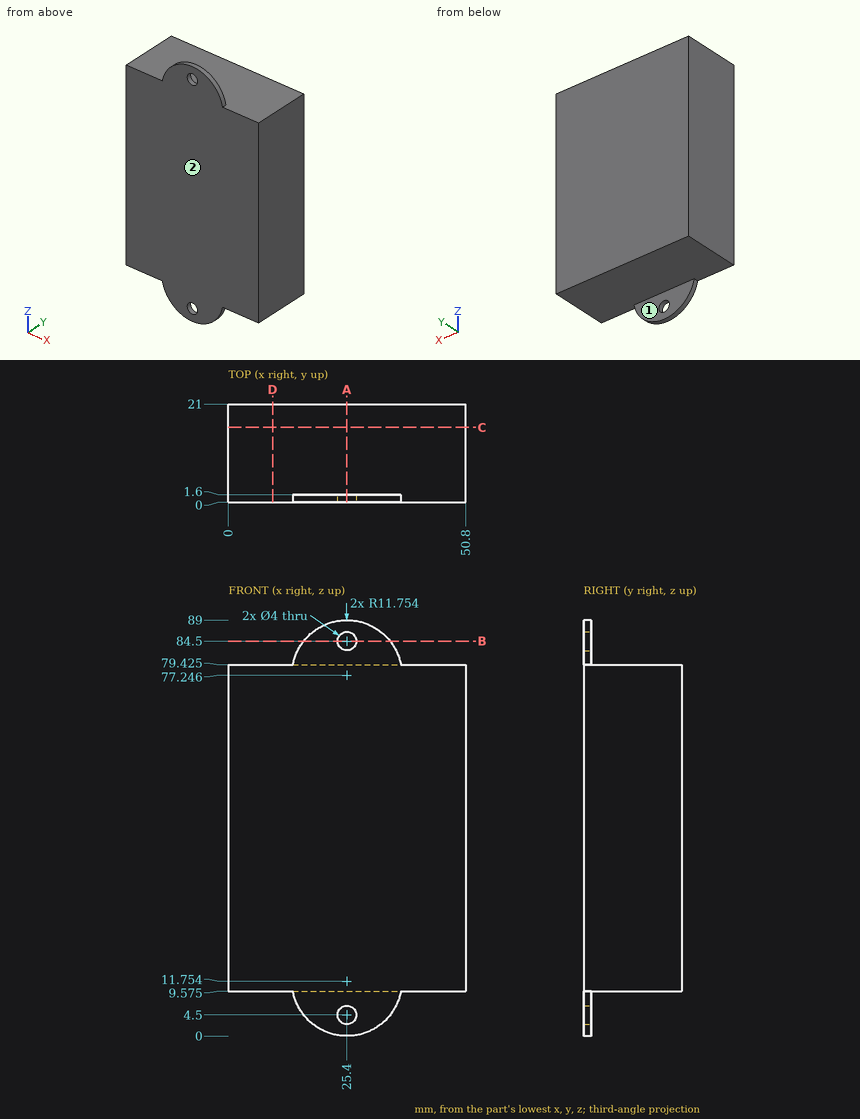
Study the drawing (mm; zero at the part's minimum x, y, z) and answer. A direction names the side the tool comes from. Coordinates: 2 decimals unless noted, no trailing zeros. Loops run counter-clockwise (first coordinate to the right, second up) from the corner with the lowest first, then second, coordinate; pieces in that order, holes last. Notation, with made-up numbers: (17.5, 68) -> (47.5, 68) arc R20 cw to (47.5, 99) -> close; hole circle Ø11 at (2, 68). An arc over 180 degrees is marked (long way). Answer as CSV lines item,"result".
1) The part is cut by section D-D (x = 9.5). Give the vertices of the cut face in (y, z) (1 decimal).
A:
outline,"(0, 9.6) -> (21, 9.6) -> (21, 79.4) -> (0, 79.4) -> close"
2) The part is cut by section C-C (y = 16). Give the vertices of the cut face in (x, z) (1 decimal).
A:
outline,"(0, 9.6) -> (50.8, 9.6) -> (50.8, 79.4) -> (0, 79.4) -> close"
3) Straight lines are drawn through the part: probe 1 along Z at (x, y) = (25.4, 0.9); probe 2 along Z at (x, y) = (46, 8) (1 decimal); probe 3 along X at (y, z) = (0.4, 84.5). For each, find the intervals that lie inside material, in ascending order.
A:
probe 1,"z = 0 to 2.5, 6.5 to 82.5, 86.5 to 89"
probe 2,"z = 9.6 to 79.4"
probe 3,"x = 16.15 to 23.4, 27.4 to 34.65"
4) The part is cut by section A-A (x = 25.4). Give the vertices of the cut face in (y, z) (1 decimal).
A:
outline,"(0, 0) -> (1.6, 0) -> (1.6, 2.5) -> (0, 2.5) -> close; (0, 6.5) -> (1.6, 6.5) -> (1.6, 9.6) -> (21, 9.6) -> (21, 79.4) -> (1.6, 79.4) -> (1.6, 82.5) -> (0, 82.5) -> close; (0, 86.5) -> (1.6, 86.5) -> (1.6, 89) -> (0, 89) -> close"
5) For the marked faces 1 and 2, determine the directions among +Z, -Z, +X, -X, +Y, -Y from which every point of the face is accessible in a straight line to the end or side of a thin tool.
A:
face 1,"-Z, +X, -X, +Y"
face 2,"+Z, -Z, +X, -X, -Y"
6) The part is cut by section B-B (z = 84.5). Give the vertices of the cut face in (x, y), and give its area (3 significant figures).
A:
outline,"(16.15, 0) -> (23.4, 0) -> (23.4, 1.6) -> (16.15, 1.6) -> close; (27.4, 0) -> (34.65, 0) -> (34.65, 1.6) -> (27.4, 1.6) -> close"
area,"23.2 mm²"
7) Flat-ended cylindrical pins translate along their axes: pin 1 (1 mm diameter, centred on x = 7.5, y = 12, fed in from +Z) (3 decimals); pin 2 (8 mm diameter, centred on x = 14.5, y = 2.5, fed in from +Z); pin 3 (5 mm diameter, centred on x = 26, z = 82.5, fed in from +Y). Find the tip coordinate at first contact, or state that the pin passes through.
A:
pin 1,"stops at z = 79.425"
pin 2,"stops at z = 86.69"
pin 3,"stops at y = 1.6"
